Could you check a few things on this model? Use its own coordinates, in mm. A direction names the side the tool comes from. Coordinates: 2 decimals unless noted, no trailing zeros. Order: outer loops, then holes, each group sorted by start corner. A loop starts at its lowest first (then second) coordinate and runs counter-clockwise, first axis right, second up. Notation, with made-up numbers: (42, -3) -> (63, -3) arc R26 ccw to (63, 26) -> close; hole circle Ø11 at (-3, 70). An arc over 180 degrees is marked (long way). Use a Markdown table: item, result. Add a question column.
1) If I drill on L1, parallel to X at y = -251.5, z = -61.5; L2, parallel to Z at x = 0, y = -91; L3, parallel to X at y = -97, z = -58, over which ranges is the centre line in solid material (lowest first)? Write a range as [from, to].
2) If we section it at A-A (y = -94): Write out the boundary of the cut face in (x, z), plus the area to 3 significant figures.
3) If we section it at B-B (y = -149.5): Write out the boundary of the cut face in (x, z).
4) Which directions (+Z, -Z, +X, -X, +Y, -Y) give clear straight access to the entire face, cutting with the end or side of a thin tool? Please do faces 1 (the flat face through (1.22, -136.396, -58.445)), 2 (the flat face through (6.22, -87.026, -67.106)), 3 (the cylindrical face through (0.257, -259.606, -56.777)).
5) Will these pins go through, and if not, where does the flat tip stop? pin 1 Ø4 at (y, z) = (-197, -66) entering from +X; pin 2 Ø5 at (x, y) = (-4.5, -80.5) entering from +Z; pin 3 Ø5 at (x, z) = (-2, -45) entering from -Y.
```python
from build123d import *

# Parameters (mm, degrees)
BOSS_EXTRUDE1_DEPTH = 4


with BuildPart() as part:
    # Sketch1 → Boss-Extrude1 (new body)
    with BuildSketch(Plane(origin=(-22.684789061, 0, -13.097069071), x_dir=(-0.5, 0, 0.866025404), z_dir=(-0.866025404, 0, -0.5))):
        with BuildLine():
            Line((-51.22508588, -207.116263928), (-51.22508588, -63.668461088))
            ThreePointArc((-51.22508588, -63.668461088), (-56.22508588, -58.668461088), (-61.22508588, -63.668461088))
            Line((-61.22508588, -63.668461088), (-61.22508588, -69.085885393))
            ThreePointArc((-61.22508588, -69.085885393), (-60.898405933, -70.181330508), (-60.02508588, -70.918915671))
            ThreePointArc((-60.02508588, -70.918915671), (-58.22508588, -73.668461088), (-60.02508588, -76.418006505))
            ThreePointArc((-60.02508588, -76.418006505), (-60.898405933, -77.155591668), (-61.22508588, -78.251036783))
            Line((-61.22508588, -78.251036783), (-61.22508588, -96.050188948))
            Line((-61.22508588, -96.050188948), (-63.318074095, -125.318595172))
            ThreePointArc((-63.318074095, -125.318595172), (-63.034364548, -126.496532456), (-62.122634264, -127.294514437))
            ThreePointArc((-62.122634264, -127.294514437), (-59.731754601, -131.246352968), (-62.660623811, -134.817775441))
            ThreePointArc((-62.660623811, -134.817775441), (-63.676623884, -135.477905129), (-64.125058417, -136.603486678))
            Line((-64.125058417, -136.603486678), (-68.745111695, -201.210442006))
            ThreePointArc((-68.745111695, -201.210442006), (-68.593140236, -207.044992568), (-67.314310613, -212.739698038))
            Line((-67.314310613, -212.739698038), (-55.328501922, -249.111405981))
            ThreePointArc((-55.328501922, -249.111405981), (-49.184106644, -259.735720996), (-39.299344022, -267.010412109))
            Line((-39.299344022, -267.010412109), (-35.743375843, -268.634553892))
            ThreePointArc((-35.743375843, -268.634553892), (-28.672308031, -268.634553892), (-28.672308031, -261.56348608))
            ThreePointArc((-28.672308031, -261.56348608), (-45.363809883, -236.582888221), (-51.22508588, -207.116263928))
        make_face()
    extrude(amount=BOSS_EXTRUDE1_DEPTH)


solid = part.part
```
Answer sheet:
| question | item | result |
|---|---|---|
| 1 | L1 | [0.64, 2.33] |
| 1 | L2 | [-60.39, -59.15] |
| 1 | L3 | [1.99, 3.24] |
| 2 | outline | (-0.54, -59.46) -> (4.46, -68.12) -> (7.93, -66.12) -> (2.93, -57.46) -> close |
| 2 | area | 40.0 mm2 |
| 3 | outline | (-0.54, -59.46) -> (6.37, -71.43) -> (9.84, -69.43) -> (2.93, -57.46) -> close |
| 4 | face 1 | +Z, -X, +Y |
| 4 | face 2 | -Z, +X, +Y |
| 4 | face 3 | -Z, +X, -Y |
| 5 | pin 1 | x = 9.01 |
| 5 | pin 2 | through |
| 5 | pin 3 | y = -268.32 |
